Solid Edge part; units mm, degrees
sketch "Sketch1" plane through (0, 0, 0) normal (-1, 0, 0) x (0, -1, 0)
  circle A0 centre (0, 0) radius 24.7
  circle A1 centre (0, 0) radius 33.5
extrude "Protrusion1" add sketch "Sketch1" along normal blind 22.5
sketch "Sketch2" plane through (-22.5, 0, 0) normal (-1, 0, 0) x (0, -1, 0)
  circle A0 centre (0, 0) radius 33.5
extrude "Protrusion2" add sketch "Sketch2" along normal blind 2
sketch "Sketch3" plane through (-24.5, 0, 0) normal (-1, 0, 0) x (0, -1, 0)
  circle A0 centre (0, 0) radius 11.4033
extrude "Cutout1" cut sketch "Sketch3" against normal up to next
sketch "Sketch4" plane through (-24.5, 0, 0) normal (-1, 0, 0) x (0, -1, 0)
  circle A0 centre (0, 0) radius 11.4033
  circle A1 centre (0, 0) radius 12.4033
extrude "Protrusion3" add sketch "Sketch4" against normal blind 11.2
sketch "Sketch5" plane through (-13.3, 0, 0) normal (1, 0, 0) x (0, 1, 0)
  circle A0 centre (0, 0) radius 1.6981
  circle A1 centre (0, 0) radius 12.4033
extrude "Protrusion4" add sketch "Sketch5" along normal blind 1.5
sketch "Sketch6" plane through (-13.3, 0, 0) normal (-1, 0, 0) x (0, -1, 0)
  circle A0 centre (0, 0) radius 1.6981
  circle A1 centre (0, 0) radius 4.875
extrude "Protrusion5" add sketch "Sketch6" along normal blind 0.5
sketch "Sketch7" plane through (-11.8, 0, 0) normal (1, 0, 0) x (0, 1, 0)
  circle A0 centre (0, 0) radius 12.4033
  circle A1 centre (0, 0) radius 10.4705
extrude "J3_Axle_BearingShoulder" add sketch "Sketch7" along normal blind 1.3
sketch "Sketch8" plane through (-10.5, 0, 0) normal (1, 0, 0) x (0, 1, 0)
  circle A0 centre (0, 0) radius 12.4033
  circle A1 centre (0, 0) radius 11.1123
extrude "J3_axle_BeaingHousing" add sketch "Sketch8" along normal blind 7.1
sketch "Sketch9" plane through (-12.25, 0, 33.5) normal (0, 0, 1) x (1, 0, 0)
  line L0 (24.75, -10) -> (-0.25, -10)
  line L1 (-0.25, -10) -> (-0.25, 10)
  line L2 (-0.25, 10) -> (24.75, 10)
  line L3 (24.75, 10) -> (24.75, -10)
extrude "Cutout2" cut sketch "Sketch9" against normal up to next
sketch "Sketch10" plane through (-11.25, 0, 24.7) normal (0, 0, 1) x (1, 0, 0)
  circle A0 centre (-7.25, 11) radius 2.1
  circle A1 centre (-7.25, -11) radius 2.1
extrude "UpperArmScrewHeadCutout" cut sketch "Sketch10" along normal mid plane 8
sketch "Sketch11" plane through (-12.25, 0, 33.5) normal (0, 0, 1) x (1, 0, 0)
  circle A0 centre (-6.25, 11) radius 1.7
  circle A1 centre (-6.25, -11) radius 1.7
extrude "UpperArmScrewCutout" cut sketch "Sketch11" against normal blind 12.8
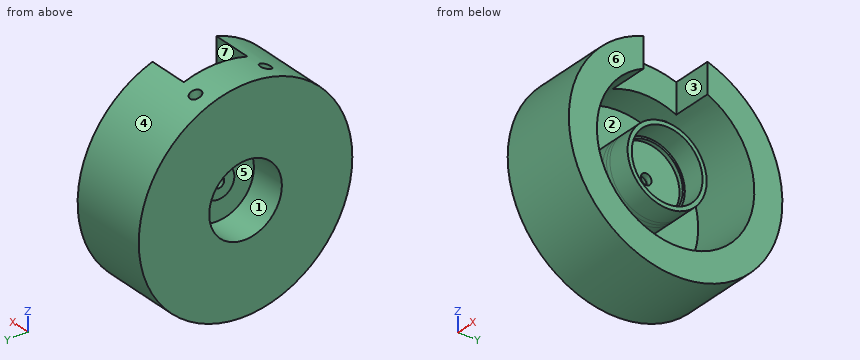
Geometry check sheet. Reference: the model listing, model coordinates, mm. Face numbers are marked on the shaded views. A direction names the side the tool comes from. Give positions to 0.01 mm unless a question says otherwise; leave off trailing zeros. Loops run counter-clockwise (first coordinate to the right, second up) from the corner with the lowest first, then second, coordinate; pieces in that order, holes last. Notation, with made-up numbers: M 13,76 L 54,76 A16 cw 54,85 Z; hole C 20.5,17.25 d1. An arc over 180 degrees is marked long. Write item = value, one per line. Start each with the question number.
1. Section check B-B, the plane x = -6. Enter the section's corners in (y, z), plus the area to 3 significant figures.
2. Section check D-D, the plane x = -15.5. Enter the section's corners in (y, z), plus the area to 3 significant figures.
3. Go/stop test with flat-tipped pins: P1, Ø4, axis at x = -3.5, y = 26, coming from the -Z side; P2, Ø2.5, axis at x = -18.5, y = 11, coming from the +Z side; P3, Ø2, axis at x = -19, y = 10.5, coming from the -Z side. Record where each tip stops, or that it passes through.
4. Thickness scan on probe 1 along Z at (x, y) = (-13.4, 0) (3 decimals); probe 2 along Z at (x, y) = (-11.3, 0); probe 3 along Y at (x, z) = (-9.5, 4). Record the ranges inside material, lowest first.
5. Draft check along Y on the marked faces 4, 5, 6 and 7. Enter one of: +Y half, -Y half, draft (parallel to the pull), parting line (faces both ways), or undercut.
6. Tool access check on the marked faces 1, 2 and 3. Record the directions out of +Z, -Z, +X, -X, +Y, -Y that give a thin tool (end or side, any length) a straight path to the whole face; none if there is none.
Values follow:
q1.outline = C 0,0 d24.81; M -10,22.59 L -10,31.97 A33.5 ccw long 10,31.97 L 10,22.59 A24.7 cw long Z; hole C 0,0 d22.22
q1.area = 1,520 mm^2
q2.outline = C 0,0 d67; C 0,0 d24.81; hole C 0,0 d49.4; hole C 0,0 d22.81
q2.area = 1,680 mm^2
q3.P1 = -23.37
q3.P2 = 7.67
q3.P3 = -32.12
q4.probe_1 = -33.5 to -24.7, -12.403 to -11.403, -4.875 to -1.698, 1.698 to 4.875, 11.403 to 12.403, 24.7 to 33.5
q4.probe_2 = -33.5 to -24.7, -12.4 to -10.47, 10.47 to 12.4
q4.probe_3 = -33.26 to -24.37, -11.74 to -10.37, 10.37 to 11.74, 24.37 to 33.26
q5.face_4 = parting line
q5.face_5 = undercut
q5.face_6 = draft
q5.face_7 = undercut
q6.face_1 = -X
q6.face_2 = +X
q6.face_3 = +Z, +X
